Geometry check sheet. Reference: the model listing, model coordinates, mm. A direction names the side the tool comes from. Coordinates: 2 decimals unless noted, no trailing zeros. Write each loop counter-clockwise with the first axis right and the second up, starting at its lowest first coordinate (ties: lowest second). Pieces come first, ordered by that corner, then holes. Notation, with made-up numbers: M 29.25,58 L 68.25,58 A21 cw 68.25,80 Z; hole C 21.5,86.5 d8. An arc over 180 degrees is marked long. Answer as a JSON object with one key per item and string values. Group by question number.
```python
from build123d import *
from OCP.BRepFilletAPI import BRepFilletAPI_MakeFillet

# Parameters (mm, degrees)
P_IDAT_VYSUNUT_M1_DEPTH       = 1
ODEBRAT_VYSUNUT_M1_DEPTH      = 65.439881064
ODEBRAT_VYSUNUT_M3_DEPTH      = 65.439881064
ODEBRAT_VYSUNUT_M3_DEPTH_BACK = 65.439881064
ODEBRAT_VYSUNUT_M4_DEPTH      = 65.439881064
ODEBRAT_VYSUNUT_M4_DEPTH_BACK = 65.439881064
ZAOBLIT1_R1                   = 2
ZAOBLIT1_R2                   = 5
ODEBRAT_VYSUNUT_M5_DEPTH      = 64.769631591
ODEBRAT_VYSUNUT_M8_DEPTH      = 64.769631591


with BuildPart() as part:
    # Skica1 → Přidat vysunutím1 (new body)
    with BuildSketch(Plane.XY):
        with BuildLine():
            Line((0, 0), (0, -20))
            ThreePointArc((0, -20), (28.666666667, -20.95661965), (57.205784047, -23.822222222))
            Line((57.205784047, -23.822222222), (59.866518188, -4))
            ThreePointArc((59.866518188, -4), (30, -1.001113587), (0, 0))
        make_face()
    extrude(amount=P_IDAT_VYSUNUT_M1_DEPTH)

    # Skica2 → Odebrat vysunutím1 (cut, through all)
    with BuildSketch(Plane.XY.offset(1)):
        with BuildLine():
            ThreePointArc((5.00678733, -7.428319839), (4.400038391, -8.021494117), (4.99321267, -8.628243057))
            ThreePointArc((4.99321267, -8.628243057), (29.426706516, -9.581983857), (53.769895868, -11.887276722))
            ThreePointArc((53.769895868, -11.887276722), (54.438517462, -11.36483518), (53.916075921, -10.696213586))
            ThreePointArc((53.916075921, -10.696213586), (29.506706624, -8.3846535), (5.00678733, -7.428319839))
        make_face()
    extrude(amount=-ODEBRAT_VYSUNUT_M1_DEPTH, mode=Mode.SUBTRACT)

    # Skica4 → Odebrat vysunutím3 (cut, two sides: drawn at the far end of the back side and taken through both)
    with BuildSketch(Plane.XY.offset(1).offset(-ODEBRAT_VYSUNUT_M3_DEPTH_BACK)):
        with BuildLine():
            Line((-132.963409192, -14), (0, -14))
            ThreePointArc((0, -14), (4.000168361, -14.018350555), (8, -14.073400674))
            Line((8, -14.073400674), (7.889908257, -20.072390573))
            Line((7.889908257, -20.072390573), (5.450212675, -153.013415352))
            Line((5.450212675, -153.013415352), (-182.994540511, -340.645096397))
            Line((-182.994540511, -340.645096397), (-321.408162378, -201.631681045))
            Line((-321.408162378, -201.631681045), (-132.963409192, -14))
        make_face()
    extrude(amount=ODEBRAT_VYSUNUT_M3_DEPTH + ODEBRAT_VYSUNUT_M3_DEPTH_BACK, mode=Mode.SUBTRACT)

    # Skica5 → Odebrat vysunutím4 (cut, two sides: drawn at the far end of the back side and taken through both)
    with BuildSketch(Plane.XY.offset(1).offset(-ODEBRAT_VYSUNUT_M4_DEPTH_BACK)):
        with BuildLine():
            Line((36.686520611, -144.697920219), (51.301744348, -23.071281094))
            Line((51.301744348, -23.071281094), (51.42105073, -22.078423608))
            Line((51.42105073, -22.078423608), (52.413908216, -22.19772999))
            ThreePointArc((52.413908216, -22.19772999), (55.198271053, -19.978877549), (52.940438573, -17.226029013))
            ThreePointArc((52.940438573, -17.226029013), (48.954265765, -16.757019834), (44.963944364, -16.324725506))
            Line((44.963944364, -16.324725506), (44.345174487, -22.292733871))
            Line((44.345174487, -22.292733871), (31.711790282, -144.141171338))
            Line((31.711790282, -144.141171338), (4.462279657, -387.624313691))
            Line((4.462279657, -387.624313691), (9.437009987, -388.181062571))
            Line((9.437009987, -388.181062571), (36.686520611, -144.697920219))
        make_face()
    extrude(amount=ODEBRAT_VYSUNUT_M4_DEPTH + ODEBRAT_VYSUNUT_M4_DEPTH_BACK, mode=Mode.SUBTRACT)

    # Zaoblit1: one fillet with a radius per group of edges: ONE call of the kernel's fillet builder (fillet() takes one radius for all edges)
    zaoblit1_edges_1 = [part.edges().sort_by_distance(p)[0] for p in [
        (0, 0, 0.5),
        (57.205784047, -23.822222222, 0.5),
        (44.345174487, -22.292733871, 0.5),
        (0, -14, 0.5),
        (7.889908257, -20.072390573, 0.5),
        (8, -14.073400674, 0.5),
        (44.963944364, -16.324725506, 0.5),
    ]]
    zaoblit1_edges_2 = [part.edges().sort_by_distance(p)[0] for p in [
        (59.866518188, -4, 0.5),
    ]]
    zaoblit1 = BRepFilletAPI_MakeFillet(part.part.solid().wrapped)
    for e in zaoblit1_edges_1:
        zaoblit1.Add(ZAOBLIT1_R1, e.wrapped)
    for e in zaoblit1_edges_2:
        zaoblit1.Add(ZAOBLIT1_R2, e.wrapped)
    add(Compound.cast(zaoblit1.Shape()), mode=Mode.REPLACE)

    # Skica6 → Odebrat vysunutím5 (cut, through all)
    with BuildSketch(Plane.XY.offset(1)):
        with BuildLine():
            ThreePointArc((47.737088512, -6.766480836), (46.77391733, -8.500998009), (46.292491489, -10.425699987))
            ThreePointArc((46.292491489, -10.425699987), (46.820211166, -11.090163638), (47.484674816, -10.562443961))
            ThreePointArc((47.484674816, -10.562443961), (47.890086051, -8.941642295), (48.701177572, -7.480996255))
            ThreePointArc((48.701177572, -7.480996255), (48.576390751, -6.641694015), (47.737088512, -6.766480836))
        make_face()
    extrude(amount=-ODEBRAT_VYSUNUT_M5_DEPTH, mode=Mode.SUBTRACT)

    # Skica7 → Odebrat vysunutím8 (cut, through all)
    with BuildSketch(Plane.XY):
        with BuildLine():
            ThreePointArc((10.533609812, -4.327670598), (9.718743083, -6.136604196), (9.399828731, -8.094802905))
            ThreePointArc((9.399828731, -8.094802905), (9.981225335, -8.712846584), (10.599269014, -8.13144998))
            ThreePointArc((10.599269014, -8.13144998), (10.867828468, -6.482440541), (11.55403203, -4.959128038))
            ThreePointArc((11.55403203, -4.959128038), (11.359549641, -4.133188209), (10.533609812, -4.327670598))
        make_face()
    extrude(amount=ODEBRAT_VYSUNUT_M8_DEPTH, mode=Mode.SUBTRACT)


solid = part.part
```
1) Section check B-B (x = 22.5). Record the cut outline in (y, z).
2) Section check C-C (y = -19.25). Record the cut outline in (x, z), then the cut area to 3 significant figures.
3) Set-up check for faces 1 (the cylindrical face through (55.192, -20.034, 0.493)), 2 (the flat face through (44.656, -19.299, 0.493)), 3 (the flat face through (29, -12, 1)): record each of +Z, -Z, +X, -X, +Y, -Y from which the full face is reachable in a straight line by a thin tool's end or side.
4) Material ranges on probe 1 along Y at (x, z) = (8.5, 0.95); probe 2 along Y at (x, z) = (19, 0.25); probe 3 along X at (y, z) = (-18, 0.1), recorded low to high. Write a range as [from, to].
5) Draft check along X on faces 4 (the cylindrical face through (53.24, -23.31, 0.49)), 5 (the flat face through (29, -12, 0)), 6 (the cylindrical face through (46.9, -8.2, 0.5)), 7 (the cylindrical face through (28.85, -0.926, 0.493)). Enter one of: +X half, -X half, draft (parallel to the pull), parting line (faces both ways), or undercut.
Entries:
{
 "1": {"outline": "M -20.59,0 L -9.17,0 L -9.17,1 L -20.59,1 Z; M -7.97,0 L -0.56,0 L -0.56,1 L -7.97,1 Z"},
 "2": {"outline": "M 8.28,0 L 44.66,0 L 44.66,1 L 8.28,1 Z; M 55.17,0 L 57.82,0 L 57.82,1 L 55.17,1 Z", "area": "39.0 mm^2"},
 "3": {"face 1": "+Z, -Z", "face 2": "+Z, -Z, -Y", "face 3": "+Z, +X, -X, +Y, -Y"},
 "4": {"probe 1": "[-19.52, -8.68], [-7.48, -0.08]", "probe 2": "[-20.42, -9.01], [-7.81, -0.4]", "probe 3": "[7.93, 44.82], [54.53, 57.99]"},
 "5": {"face 4": "-X half", "face 5": "draft", "face 6": "undercut", "face 7": "+X half"}
}
